from build123d import *

# Parameters (mm, degrees)
F0_R     = 2.15
F0_R_2   = 3
F0_R_3   = 1.5
F0_R_4   = 5
F1_DEPTH = 5
F2_R     = 1
F3_R     = 5
F4_DEPTH = 7
F6_W     = 20.916191861
F6_H     = 23.5347189009
F6_W_2   = 37.2305270284
F6_H_2   = 26.8968194723
F7_DEPTH = 25
F8_R     = 5


# Not quite as in the source:
# - a fillet or chamfer that OpenCascade refuses, or shapes differently, is made with other operations: its cross-section is extruded or revolved along the edge and cut away or added


with BuildPart() as f1:
    # F0 (on Top) → F1 (new body)
    with BuildSketch(Plane.XY):
        Polygon((-49.7560231508, 20), (-49.7560231508, 0), (76.2439768492, 0), (76.2439768492, 20), (33.2439768492, 20), (-6.7560231508, 20), align=None)
        with Locations((-45.6060231508, 9.15)):
            Circle(F0_R, mode=Mode.SUBTRACT)
        with Locations((72.0939768492, 9.15)):
            Circle(F0_R, mode=Mode.SUBTRACT)
        Polygon((-49.7560231508, 106.5), (-49.7560231508, 20), (-6.7560231508, 20), (-6.7560231508, 25), (33.2439768492, 25), (33.2439768492, 20), (76.2439768492, 20), (76.2439768492, 106.5), (33.2439768492, 106.5), (33.2439768492, 101.5), (-6.7560231508, 101.5), (-6.7560231508, 106.5), align=None)
        with Locations((-34.7560231508, 39.25)):
            Circle(F0_R_2, mode=Mode.SUBTRACT)
        with Locations((3.2439768492, 53.25)):
            Circle(F0_R_3, mode=Mode.SUBTRACT)
        with Locations((23.2439768492, 53.25)):
            Circle(F0_R_3, mode=Mode.SUBTRACT)
        with Locations((48.2439768492, 39.25)):
            Circle(F0_R_2, mode=Mode.SUBTRACT)
        with Locations((3.2439768492, 73.25)):
            Circle(F0_R_3, mode=Mode.SUBTRACT)
        with Locations((-34.7560231508, 87.25)):
            Circle(F0_R_2, mode=Mode.SUBTRACT)
        with Locations((13.2439768492, 63.25)):
            Circle(F0_R_4, mode=Mode.SUBTRACT)
        with Locations((23.2439768492, 73.25)):
            Circle(F0_R_3, mode=Mode.SUBTRACT)
        with Locations((48.2439768492, 87.25)):
            Circle(F0_R_2, mode=Mode.SUBTRACT)
        Polygon((-49.7560231508, 111.5), (-49.7560231508, 106.5), (-6.7560231508, 106.5), (33.2439768492, 106.5), (76.2439768492, 106.5), (76.2439768492, 111.5), align=None)
        with Locations((-34.7560231508, 39.25)):
            Circle(F0_R_2)
        with Locations((-34.7560231508, 39.25)):
            Circle(F0_R_3, mode=Mode.SUBTRACT)
        with Locations((-34.7560231508, 87.25)):
            Circle(F0_R_2)
        with Locations((-34.7560231508, 87.25)):
            Circle(F0_R_3, mode=Mode.SUBTRACT)
        with Locations((48.2439768492, 39.25)):
            Circle(F0_R_2)
        with Locations((48.2439768492, 39.25)):
            Circle(F0_R_3, mode=Mode.SUBTRACT)
        with Locations((48.2439768492, 87.25)):
            Circle(F0_R_2)
        with Locations((48.2439768492, 87.25)):
            Circle(F0_R_3, mode=Mode.SUBTRACT)
        with Locations((13.2439768492, 63.25)):
            Circle(F0_R_4)
        with Locations((3.2439768492, 73.25)):
            Circle(F0_R_3)
        with Locations((3.2439768492, 53.25)):
            Circle(F0_R_3)
        with Locations((23.2439768492, 53.25)):
            Circle(F0_R_3)
        with Locations((23.2439768492, 73.25)):
            Circle(F0_R_3)
    extrude(amount=F1_DEPTH)

    # F2
    f2_edges = [f1.edges().sort_by_distance(p)[0] for p in [
        (-6.756023, 25, 2.5),
        (33.243977, 25, 2.5),
        (-6.756023, 20, 2.5),
        (33.243977, 20, 2.5),
        (-6.756023, 101.5, 2.5),
        (-6.756023, 106.5, 2.5),
        (33.243977, 106.5, 2.5),
        (33.243977, 101.5, 2.5),
    ]]
    fillet(f2_edges, radius=F2_R)

    # F3
    f3_edges = [f1.edges().sort_by_distance(p)[0] for p in [
        (-49.756023, 0, 2.5),
        (76.243977, 0, 2.5),
        (76.243977, 111.5, 2.5),
        (-49.756023, 111.5, 2.5),
    ]]
    fillet(f3_edges, radius=F3_R)

    # F0 (on Top) → F4 (join)
    with BuildSketch(Plane.XY):
        with Locations((-34.7560231508, 87.25)):
            Circle(F0_R_2)
        with Locations((-34.7560231508, 87.25)):
            Circle(F0_R_3, mode=Mode.SUBTRACT)
        with Locations((-34.7560231508, 39.25)):
            Circle(F0_R_2)
        with Locations((-34.7560231508, 39.25)):
            Circle(F0_R_3, mode=Mode.SUBTRACT)
        with Locations((48.2439768492, 87.25)):
            Circle(F0_R_2)
        with Locations((48.2439768492, 87.25)):
            Circle(F0_R_3, mode=Mode.SUBTRACT)
        with Locations((48.2439768492, 39.25)):
            Circle(F0_R_2)
        with Locations((48.2439768492, 39.25)):
            Circle(F0_R_3, mode=Mode.SUBTRACT)
    extrude(amount=F4_DEPTH)

    # F5: fillet of radius 5 on 4 edges, made by hand

    # F5_s1 → F5_t2 (revolve)
    with BuildSketch(Plane.XZ.offset(-87.25)):
        with BuildLine():
            ThreePointArc((-27.7560231508, 5), (-29.9920911283, 5.527864045), (-31.7560231508, 7))
            Line((-31.7560231508, 7), (-31.7560231508, 5))
            Line((-31.7560231508, 5), (-27.7560231508, 5))
        make_face()
    revolve(axis=Axis((-34.7560231508, 87.25, 5), (0, 0, -1)))

    # F5_s3 → F5_t4 (revolve)
    with BuildSketch(Plane.XZ.offset(-39.25)):
        with BuildLine():
            ThreePointArc((-27.7560231508, 5), (-29.9920911283, 5.527864045), (-31.7560231508, 7))
            Line((-31.7560231508, 7), (-31.7560231508, 5))
            Line((-31.7560231508, 5), (-27.7560231508, 5))
        make_face()
    revolve(axis=Axis((-34.7560231508, 39.25, 5), (0, 0, -1)))

    # F5_s5 → F5_t6 (revolve)
    with BuildSketch(Plane.XZ.offset(-39.25)):
        with BuildLine():
            ThreePointArc((55.2439768492, 5), (53.0079088717, 5.527864045), (51.2439768492, 7))
            Line((51.2439768492, 7), (51.2439768492, 5))
            Line((51.2439768492, 5), (55.2439768492, 5))
        make_face()
    revolve(axis=Axis((48.2439768492, 39.25, 5), (0, 0, -1)))

    # F5_s7 → F5_t8 (revolve)
    with BuildSketch(Plane.XZ.offset(-87.25)):
        with BuildLine():
            ThreePointArc((51.2439768492, 7), (53.0079088717, 5.527864045), (55.2439768492, 5))
            Line((55.2439768492, 5), (51.2439768492, 5))
            Line((51.2439768492, 5), (51.2439768492, 7))
        make_face()
    revolve(axis=Axis((48.2439768492, 87.25, 5), (0, 0, -1)))

    # F6 (on face) → F7 (cut)
    with BuildSketch(Plane.XY.offset(5)):
        Polygon((33.4173643496, 97.5044071674), (-20.9036788438, 97.5044071674), (-20.9036788438, 74.5087079704), (-20.9036788438, 50.9739890695), (-20.9036788438, 28.7407264113), (33.4173643496, 28.7407264113), (33.4173643496, 49.8894378543), (33.4173643496, 76.7862573266), align=None)
        with Locations((-31.3617747743, 62.7413485199)):
            Rectangle(F6_W, F6_H)
        with Locations((52.0326278638, 63.3378475904)):
            Rectangle(F6_W_2, F6_H_2)
    extrude(amount=-F7_DEPTH, mode=Mode.SUBTRACT)

    # F8
    f8_edges = [f1.edges().sort_by_distance(p)[0] for p in [
        (-20.903679, 74.508708, 2.5),
        (33.417364, 76.786257, 2.5),
        (33.417364, 49.889438, 2.5),
        (-20.903679, 50.973989, 2.5),
        (-41.819871, 50.973989, 2.5),
        (-41.819871, 74.508708, 2.5),
        (-20.903679, 97.504407, 2.5),
        (33.417364, 97.504407, 2.5),
        (70.647891, 76.786257, 2.5),
        (70.647891, 49.889438, 2.5),
        (33.417364, 28.740726, 2.5),
        (-20.903679, 28.740726, 2.5),
    ]]
    fillet(f8_edges, radius=F8_R)


solid = f1.part
Geometry: final body of the model. Coordinates: model frame, mm. A direction names the side the tool comes from. Give positions to 0.01 mm unless a question says otherwise; leave off trailing zeros. Write each loop counter-clockwise with the first axis right and the second up, starting at its lowest first coordinate (ties: lowest second). Pieces come first, ordered by that corner, then holes. Notation, with made-up numbers: M 48,-20 L 93,-20 A30 ccw 93,17 Z; hole C -8.5,-19.75 d2. An arc over 180 degrees is marked long. Answer in a Markdown table with one row per item. Add a question column.
(1) Section A-A on y = 87.25. Return loops of the section in (x, z), and give its area (3 significant figures).
(2) Mould query, pull axis Y, two halves, no side actions, for faces 3 (the flat face through (40, 44, 0)), 4 (the cylindrical face through (69.144, 51.315, 2.465)), 5 (the flat face through (12, 0, 2)), 6 (the flat face through (14, 111.5, 2)). Classes: +Y half, -Y half, draft (parallel to the pull), parting line (faces both ways), or undercut.
(3) Reachability of faces 1 (the flat face through (-31, 74.509, 3)), 2 (the flat face through (-34, 41, 7)) from +Z, -Z, +X, -X, +Y, -Y: full face, straight path, thin tool, end or side. Return the list, or none.
(4) Section C-C on x = 30. Return loops of the section in (y, z), and give its area (3 significant figures).
(5) First-contact query: pin 1 (4 mm diameter, centred on x = -45.61, y = 9.15, fed in from +Z); pin 2 (8 mm diameter, centred on x = -30.5, y = 97.5, fed in from +Z); pin 3 (3.5 mm diameter, centred on x = 48.24, y = 39.25, fed in from -Z). Flat tips, straight axial feed; report the tip coordinate or a pass-through.
(6) Section B-B on y = 9.15. Return loops of the section in (x, z), and give its area (3 significant figures).
(7) Section D-D on z = 3. State how many separate pieces and enclosed holes the cut face has, and give its area (3 significant figures).
(8) Ray query, line 1 (X direction, y = 87, z = 3.75); line 2 (X direction, y = 61, z = 3); line 3 (X direction, y = 87.25, z = 2). Return the intervals inside material, ascending.
Result set:
| question | item | result |
|---|---|---|
| 1 | outline | M -49.76,0 L -36.26,0 L -36.26,7 L -37.76,7 A5 cw -41.76,5 L -49.76,5 Z; M -33.26,0 L -20.9,0 L -20.9,5 L -27.76,5 A5 cw -31.76,7 L -33.26,7 Z; M 33.42,0 L 46.74,0 L 46.74,7 L 45.24,7 A5 cw 41.24,5 L 33.42,5 Z; M 49.74,0 L 76.24,0 L 76.24,5 L 55.24,5 A5 cw 51.24,7 L 49.74,7 Z |
| 1 | area | 350 mm^2 |
| 2 | face 3 | draft |
| 2 | face 4 | undercut |
| 2 | face 5 | -Y half |
| 2 | face 6 | +Y half |
| 3 | face 1 | +Z, -Z |
| 3 | face 2 | +Z, +X, -X, +Y, -Y |
| 4 | outline | M 0,0 L 20,0 L 20,5 L 0,5 Z; M 25,0 L 29,0 L 29,5 L 25,5 Z; M 97.25,0 L 101.5,0 L 101.5,5 L 97.25,5 Z; M 106.5,0 L 111.5,0 L 111.5,5 L 106.5,5 Z |
| 4 | area | 166 mm^2 |
| 5 | pin 1 | passes through |
| 5 | pin 2 | stops at z = 5 |
| 5 | pin 3 | stops at z = 0 |
| 6 | outline | M -49.76,0 L -47.76,0 L -47.76,5 L -49.76,5 Z; M -43.46,0 L 69.94,0 L 69.94,5 L -43.46,5 Z; M 74.24,0 L 76.24,0 L 76.24,5 L 74.24,5 Z |
| 6 | area | 587 mm^2 |
| 7 | separate pieces | 1 |
| 7 | enclosed holes | 9 |
| 7 | area | 8,360 mm^2 |
| 8 | line 1 | x = -49.76 to -36.24, -33.28 to -20.9, 33.42 to 46.76, 49.72 to 76.24 |
| 8 | line 2 | x = -49.76 to -41.82, 70.65 to 76.24 |
| 8 | line 3 | x = -49.76 to -36.26, -33.26 to -20.9, 33.42 to 46.74, 49.74 to 76.24 |
